```python
from build123d import *

# Parameters (mm, degrees)
F0_R     = 22.225
F1_DEPTH = 44.45
F2_R     = 7.9375
F3_DEPTH = 9.525


with BuildPart() as f1:
    # F0 (on Right) → F1 (new body, symmetric)
    with BuildSketch(Plane.YZ):
        Circle(F0_R)
    extrude(amount=F1_DEPTH, both=True)

    # F2 (on face) → F3 (join)
    with BuildSketch(Plane(origin=(-44.45, 0, 0), x_dir=(0, -1, 0), z_dir=(-1, 0, 0))):
        with BuildLine():
            Line((-22.225, 76.2), (-22.225, 0))
            ThreePointArc((-22.225, 0), (0, -22.225), (22.225, 0))
            Line((22.225, 0), (22.225, 76.2))
            ThreePointArc((22.225, 76.2), (0, 98.425), (-22.225, 76.2))
        make_face()
        Circle(F2_R, mode=Mode.SUBTRACT)
        with Locations((0, 76.2)):
            Circle(F2_R, mode=Mode.SUBTRACT)
    extrude(amount=F3_DEPTH)

    # F4: F1 across plane


with BuildPart() as f1_1:
    add(f1.part)
    add(f1.part.mirror(Plane.YZ))


solid = f1_1.part
```
Verification items for the finished model (mm, model axes). A direction names the side the tool comes from. Give positions to 0.01 mm unless a question says otherwise; leave off trailing zeros. Order: outer loops, then holes, each group sorted by start corner. A loop starts at its lowest first (then second) coordinate and runs counter-clockwise, first axis right, second up. Notation, with made-up numbers: M -2,-23 L 38,-23 A24 cw 38,7 Z; hole C 2.25,42 d6. An arc over 180 degrees is marked long. Return JSON: item names as keys, results as strings. Group by question number.
1) Section check C-C on x = 7. Record the cut outline in (y, z) (3 decimals).
2) Section check A-A on z = 38.5. Record the cut outline in (x, y) (3 decimals), and give its area (3 significant figures).
3) Scan lines: line 1 (Z direction, x = -47.25, y = 0) (1 decimal); line 2 (X direction, y = -18.5, z = 44.5) (3 decimals); line 3 (Y direction, x = 19, z = 13). Record each from-to range of solid material in increasing order.
4) Section check D-D on y = 15.5. Record the cut outline in (x, z) (3 decimals).
5) Access from +Z, -Z, +X, -X, +Y, -Y to the whole of each face (thin tool, end or side, straight path). Record for faces 5 (the face through (49.15, 1.03, 84.07)), 6 (the face through (49.15, 1.72, -7.75)), 7 (the face through (-49.15, 1.72, -7.75)).
6) Go/stop test with flat-tipped pins: pin 1 Ø12.5 at (y, z) = (0, 76.2) entering from +X; pin 2 Ø4 at (x, y) = (37.5, -14) entering from -Z; pin 3 Ø10 at (x, y) = (4.5, -11) entering from -Z; pin 4 Ø3 at (x, y) = (-7.5, -3) entering from -Z. Record where each tip stops, or that it passes through.
7) Section check B-B on y = 0. Give the number of separate pieces and of enclosed holes in the cut face, and give its area (3 significant figures).
8) Mould release check, pull along Z, two halves, no side actions. Record for faces 1 (the face through (44.45, 0, 0)), 2 (the face through (-49.15, -0.49, 98.42)), 3 (the face through (-0.756, -2.893, -22.036)), 4 (the face through (-44.45, 0, 50)): pulls with the +Z half, pulls with the -Z half, needs draft (parallel to the pull), parting line crosses it, or undercut.
Answer block:
{
 "1": {"outline": "C 0,0 d44.45"},
 "2": {"outline": "M -53.975,-22.225 L -44.45,-22.225 L -44.45,22.225 L -53.975,22.225 Z; M 44.45,-22.225 L 53.975,-22.225 L 53.975,22.225 L 44.45,22.225 Z", "area": "847 mm^2"},
 "3": {"line 1": "z = -22.2 to -7.9, 7.9 to 68.3, 84.1 to 98.4", "line 2": "x = -53.975 to -44.45, 44.45 to 53.975", "line 3": "y = -18.03 to 18.03"},
 "4": {"outline": "M -53.975,-15.928 L 53.975,-15.928 L 53.975,92.128 L 44.45,92.128 L 44.45,15.928 L -44.45,15.928 L -44.45,92.128 L -53.975,92.128 Z"},
 "5": {"face 5": "+X, -X", "face 6": "+X", "face 7": "-X"},
 "6": {"pin 1": "passes through", "pin 2": "stops at z = -18.71", "pin 3": "stops at z = -21.4", "pin 4": "stops at z = -22.17"},
 "7": {"separate pieces": "3", "enclosed holes": "0", "area": "5,650 mm^2"},
 "8": {"face 1": "undercut", "face 2": "pulls with the +Z half", "face 3": "parting line crosses it", "face 4": "needs draft"}
}
